```python
from build123d import *

# Parameters (mm, degrees)
F0_W     = 60
F0_H     = 60
F0_R     = 2
F1_DEPTH = 1
F2_R     = 5


with BuildPart() as f1:
    # F0 (on Top) → F1 (new body)
    with BuildSketch(Plane.XY):
        Rectangle(F0_W, F0_H)
        with Locations((-25, -25)):
            Circle(F0_R, mode=Mode.SUBTRACT)
        with BuildLine():
            Line((-23.561762, -14.18074), (-17.931378, -10.930036))
            ThreePointArc((-17.931378, -10.930036), (0, -21), (17.931378, -10.930036))
            Line((17.931378, -10.930036), (23.561762, -14.18074))
            ThreePointArc((23.561762, -14.18074), (0, -27.5), (-23.561762, -14.18074))
        make_face(mode=Mode.SUBTRACT)
        with Locations((25, -25)):
            Circle(F0_R, mode=Mode.SUBTRACT)
        with BuildLine():
            ThreePointArc((17.065095, -10.429887), (0, -20), (-17.065095, -10.429887))
            Line((-17.065095, -10.429887), (-8.399422, -5.426759))
            ThreePointArc((-8.399422, -5.426759), (0, -10), (8.399422, -5.426759))
            Line((8.399422, -5.426759), (17.065095, -10.429887))
        make_face(mode=Mode.SUBTRACT)
        with BuildLine():
            ThreePointArc((-24.061762, -13.314714), (-23.815699, 13.75), (-0.5, 27.495454))
            Line((-0.5, 27.495454), (-0.5, 20.994047))
            ThreePointArc((-0.5, 20.994047), (-18.186533, 10.5), (-18.431378, -10.064011))
            Line((-18.431378, -10.064011), (-24.061762, -13.314714))
        make_face(mode=Mode.SUBTRACT)
        with BuildLine():
            Line((-0.5, 19.993749), (-0.5, 9.987492))
            ThreePointArc((-0.5, 9.987492), (-8.660254, 5), (-8.899422, -4.560733))
            Line((-8.899422, -4.560733), (-17.565095, -9.563862))
            ThreePointArc((-17.565095, -9.563862), (-17.320508, 10), (-0.5, 19.993749))
        make_face(mode=Mode.SUBTRACT)
        with Locations((-25, 25)):
            Circle(F0_R, mode=Mode.SUBTRACT)
        with BuildLine():
            Line((17.565095, -9.563862), (8.899422, -4.560733))
            ThreePointArc((8.899422, -4.560733), (8.660254, 5), (0.5, 9.987492))
            Line((0.5, 9.987492), (0.5, 19.993749))
            ThreePointArc((0.5, 19.993749), (17.320508, 10), (17.565095, -9.563862))
        make_face(mode=Mode.SUBTRACT)
        with BuildLine():
            Line((24.061762, -13.314714), (18.431378, -10.064011))
            ThreePointArc((18.431378, -10.064011), (18.186533, 10.5), (0.5, 20.994047))
            Line((0.5, 20.994047), (0.5, 27.495454))
            ThreePointArc((0.5, 27.495454), (23.815699, 13.75), (24.061762, -13.314714))
        make_face(mode=Mode.SUBTRACT)
        with Locations((25, 25)):
            Circle(F0_R, mode=Mode.SUBTRACT)
    extrude(amount=F1_DEPTH)

    # F2
    f2_edges = [f1.edges().sort_by_distance(p)[0] for p in [
        (-30, -30, 0.5),
        (30, -30, 0.5),
        (-30, 30, 0.5),
        (30, 30, 0.5),
    ]]
    fillet(f2_edges, radius=F2_R)


solid = f1.part
```
Geometry check sheet. Reference: the model listing, model coordinates, mm. Give positions to 0.01 mm unless a question says otherwise; leave off trailing zeros. Loops run counter-clockwise (first coordinate to the right, second up) from the corner with the lowest first, then second, coordinate; pieces in that order, holes last. Notation, with made-up numbers: M -22,30 L 17,30 A23 cw 17,46 Z; hole C -1,47 d6. An arc over 180 degrees is marked long. Answer as CSV lines item,"result".
Item 1: Cross-section at B-B on z = 0.2. Count the separate pieces of the cut face and the enclosed holes in it, and give its area (3 significant figures).
Values:
separate pieces,"1"
enclosed holes,"10"
area,"1,640 mm²"
Item 2: Cross-section at D-D on x = -3.5. Record the cut outline in (y, z).
Values:
outline,"M -30,0 L -27.28,0 L -27.28,1 L -30,1 Z; M -20.71,0 L -19.69,0 L -19.69,1 L -20.71,1 Z; M -9.37,0 L 9.37,0 L 9.37,1 L -9.37,1 Z; M 19.69,0 L 20.71,0 L 20.71,1 L 19.69,1 Z; M 27.28,0 L 30,0 L 30,1 L 27.28,1 Z"
Item 3: Cross-section at C-C on x = 22. Record the cut outline in (y, z), and give its area (3 significant figures).
Values:
outline,"M -30,0 L -16.5,0 L -16.5,1 L -30,1 Z; M -13.28,0 L -12.12,0 L -12.12,1 L -13.28,1 Z; M 16.5,0 L 30,0 L 30,1 L 16.5,1 Z"
area,"28.2 mm²"
Item 4: Cross-section at A-A on x = 5. Record the cut outline in (y, z).
Values:
outline,"M -30,0 L -27.04,0 L -27.04,1 L -30,1 Z; M -20.4,0 L -19.36,0 L -19.36,1 L -20.4,1 Z; M -8.66,0 L 8.66,0 L 8.66,1 L -8.66,1 Z; M 19.36,0 L 20.4,0 L 20.4,1 L 19.36,1 Z; M 27.04,0 L 30,0 L 30,1 L 27.04,1 Z"
Item 5: Depth check by flat-ended pin: P1, Ø4.5, axis at x = -25, y = -25, coming from the +Z side. Enter the tip coordinate at first touch or a pass-through.
Values:
P1,"stops at z = 1"
Item 6: Release check for a two-part mould opening along X. For faces 1 (the cylindrical face through (-28.57, -28.5, 0.51)), 2 (the cylindrical face through (-26.6, -26.2, 0.5)), 3 (the cylindrical face through (28.5, 28.57, 0.51)) record: pulls with the +X half, pulls with the -X half, needs draft (parallel to the pull), parting line crosses it, or undercut.
Values:
face 1,"pulls with the -X half"
face 2,"undercut"
face 3,"pulls with the +X half"
Item 7: Material ranges on line 1 (X direction, y = 0, z = 0.35); line 2 (Y direction, x = 9, z = 0.15); line 3 (Y direction, x = 25, z = 0.6), recorded low to high.
Values:
line 1,"x = -30 to -27.5, -21 to -20, -10 to 10, 20 to 21, 27.5 to 30"
line 2,"y = -30 to -25.99, -18.97 to -17.86, -5.77 to -4.62, -4.36 to 4.36, 17.86 to 18.97, 25.99 to 30"
line 3,"y = -30 to -27, -23 to -11.46, 11.46 to 23, 27 to 30"
